Input: dimensioned drawing with shaded views. Units: mm. Origin: part minimum x, y, z. Round coordinates to 2 decimals unless told otherwise and drop trailing zeros. Loops run counter-clockwise (first coordinate to the right, second up) from the corner with the lowest first, then second, coordinate; pieces in that order, holes last. Notation, with made-up numbers: (55.25, 74) - (112.25, 74) arc R15 ccw to (112.25, 85) - close; hole circle Ø6 at (35.5, 41). An arc over 180 degrees is marked (long way). One line per question, with ' | ' between items. Start each with the question number.
Item 1: Section D-D, the plane z = 67.75. Return loops of the section in (x, y), plus the area to 3 significant figures.
Item 2: Section B-B, the plane x = 56.25. Return loops of the section in (y, z), plus the area to 3 significant figures.
Item 3: Material intervals for line 1 along X through (y, z) = (1.2, 67.75); line 2 along X through (y, z) = (2.25, 18.75); line 3 along Z through (x, y) = (9.25, 1.2), sorted ascending.
Item 4: Section C-C, the plane y = 2.8. Return loops of the section in (x, z).
Item 5: Section A-A, the plane z = 18.75. Return loops of the section in (x, y), plus the area to 3 significant figures.
Item 6: First-contact query: pin 1 (1 mm diameter, centred on x = 26.5, z = 29, fed in from -Y); pin 2 (0.6 mm diameter, centred on y = 3, z = 31.5, fed in from -X); pin 3 (0.9 mm diameter, centred on x = 62.5, z = 44, fed in from +Y); pin 4 (1.6 mm diameter, centred on y = 3.5, z = 44.5, fed in from +X). Flat tips, straight axial feed; report the tip coordinate or a pass-through.
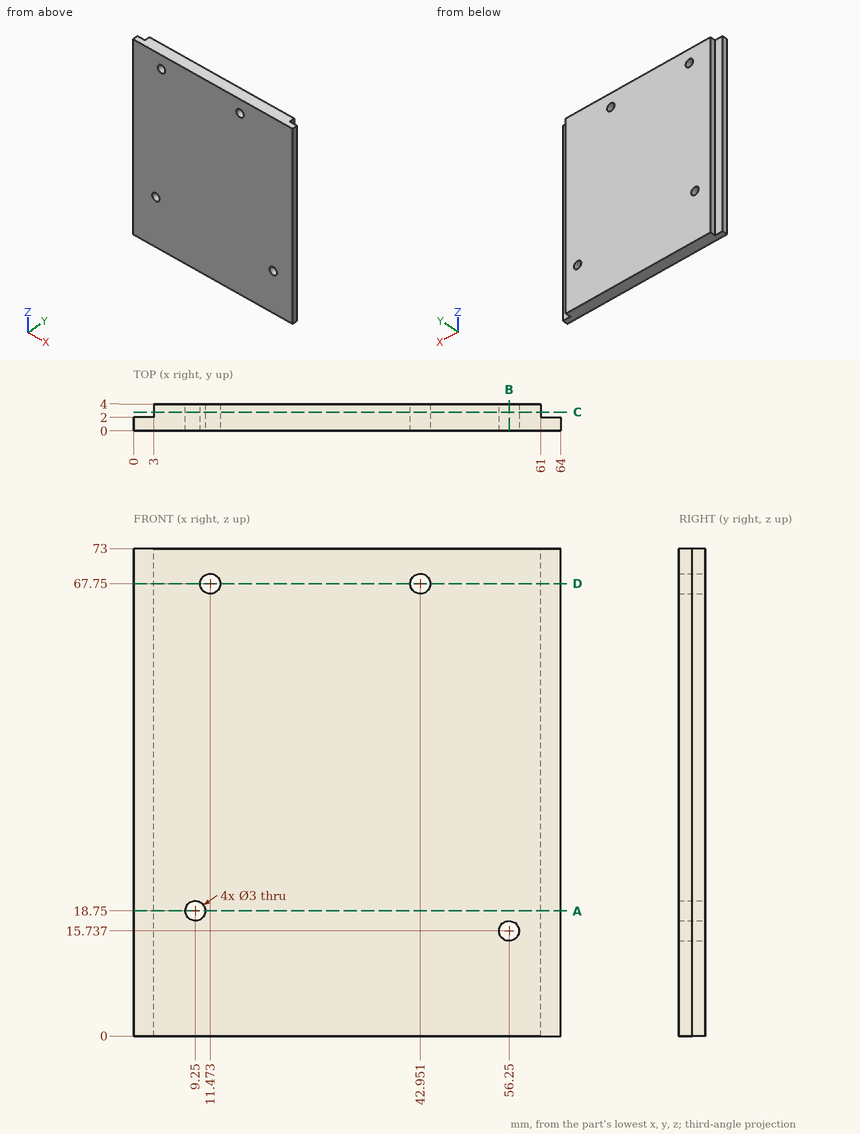
Return value:
1) outline: (0, 0) - (9.97, 0) - (9.97, 4) - (3, 4) - (3, 2) - (0, 2) - close; (12.97, 0) - (41.45, 0) - (41.45, 4) - (12.97, 4) - close; (44.45, 0) - (64, 0) - (64, 2) - (61, 2) - (61, 4) - (44.45, 4) - close | area: 220 mm2
2) outline: (0, 0) - (4, 0) - (4, 14.24) - (0, 14.24) - close; (0, 17.24) - (4, 17.24) - (4, 73) - (0, 73) - close | area: 280 mm2
3) line 1: 0 to 9.97, 12.97 to 41.45, 44.45 to 64 | line 2: 3 to 7.75, 10.75 to 61 | line 3: 0 to 17.25, 20.25 to 73
4) outline: (3, 0) - (61, 0) - (61, 73) - (3, 73) - close; hole circle Ø3 at (9.25, 18.75); hole circle Ø3 at (11.47, 67.75); hole circle Ø3 at (42.95, 67.75); hole circle Ø3 at (56.25, 15.74)
5) outline: (0, 0) - (7.75, 0) - (7.75, 4) - (3, 4) - (3, 2) - (0, 2) - close; (10.75, 0) - (64, 0) - (64, 2) - (61, 2) - (61, 4) - (10.75, 4) - close | area: 232 mm2
6) pin 1: y = 0 | pin 2: x = 3 | pin 3: y = 2 | pin 4: x = 61
